Work out the finished part from the listing and answer in its coordinate system (mm). Face numbers are marked on the shaded views. A direction names the side the tool comes from. Round coordinates to 2 decimals unless told otherwise and drop trailing zeros. Order: outer loops, then holes, each group sorted by start corner. A loop starts at its lowest first (then second) coordinate and runs counter-clockwise, first axis right, second up. Notation, with made-up numbers: M 67,80 L 101,80 A26 cw 101,100 Z; hole C 68.5,-3.75 d3. An arc over 180 degrees is marked long. Answer as a JSON object with one key per item and string values. Group by question number.
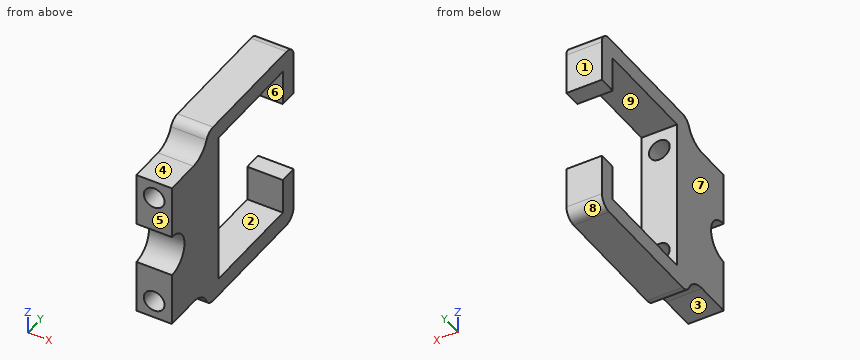
Autodesk Inventor part; units mm, degrees
ref_plane "YZ Plane" through (0, 0, 0) normal (1, 0, 0) x (0, 1, 0)
ref_plane "XZ Plane" through (0, 0, 0) normal (0, 1, 0) x (-1, 0, 0)
ref_plane "XY Plane" through (0, 0, 0) normal (0, 0, 1) x (1, 0, 0)
sketch "Esquisse1" plane through (0, 0, 0) normal (1, 0, 0) x (0, 1, 0)
  arc A0 (0, -3.5) -> (0, 3.5) centre (0, 0) ccw
  line L0 (0, 6.2947) -> (0, -6.5718) construction
  line L1 (0, 3.5) -> (0, 12.5)
  line L2 (0, 12.5) -> (10, 12.5)
  line L3 (10, -12.5) -> (0, -12.5)
  line L4 (0, -12.5) -> (0, -3.5)
  line L5 (10, 12.5) -> (10, 16)
  line L6 (10, 16) -> (34, 16)
  line L7 (34, 16) -> (34, 7)
  line L8 (34, 7) -> (31, 7)
  line L9 (31, 7) -> (31, 13)
  line L10 (31, 13) -> (13, 13)
  line L11 (13, 13) -> (13, -13)
  line L12 (13, -13) -> (31, -13)
  line L13 (31, -13) -> (31, -7)
  line L14 (31, -7) -> (34, -7)
  line L15 (34, -7) -> (34, -16)
  line L16 (34, -16) -> (10, -16)
  line L17 (10, -16) -> (10, -12.5)
  point P0 (22, 13)
  dimension "d16" = 3.5
  dimension "d17" = 25
  dimension "d18" = 26
  dimension "d19" = 6
  dimension "d20" = 3
  dimension "d21" = 3
  dimension "d22" = 3
  dimension "d23" = 18
  dimension "d24" = 3
  dimension "d25" = 10
extrude "Extrusion1" add sketch "Esquisse1" along normal blind 6
fillet "Congé1" radius 4 2 edges at (3, 10, 12.5) (3, 10, -12.5)
fillet "Congé2" radius 2 2 edges at (3, 10, -16) (3, 10, 16)
fillet "Congé3" radius 2 2 edges at (3, 34, 16) (3, 34, -16)
sketch "Esquisse2" plane through (0, 0, -12.5) normal (0, -1, 0) x (1, 0, 0)
  circle A0 centre (3, 3) radius 1.75
  line L0 (0, -1.5) -> (0, 5.5)
  line L1 (6, -0.5) -> (6, 25.5)
  line L2 (0, -0.5) -> (0, 25.5)
  line L3 (0, 0) -> (6, 0)
  point P0 (0, 12.5)
  point P1 (3, 3)
  dimension "d28" = 3.5
  dimension "d31" = 3
  dimension "d32" = 3
extrude "Extrusion2" cut sketch "Esquisse2" against normal blind 15
mirror "Mise en miroir1" about plane through (0, 0, 0) normal (0, 0, 1) of "Extrusion2"
properties part number "Bras_1_Impression 3D"
Item 1: Each of these flat-tipped pins is pushed along its axis until it touches: pin 1 (1.8 mm diameter, centred on x = 3.5, y = 4, fed in from +Z); pin 2 (1.5 mm diameter, centred on x = 2, y = 33, fed in from +Z); pin 3 (1.8 mm diameter, centred on x = 3, y = 1.5, fed in from -Z). Where does it stop, or does it pass through?
Item 2: Consider L1, parallel to Z at x = 3, y = 6; L2, parallel to Z at x = 3.45, y = 14.5; L3, parallel to X at y = 5.25, z = 9.5. Determine where each line is inside the solid, lowest interval first.
Item 3: Find section A-A (z = -9.5). Give the vertices of the cut face in (x, y), and give its area (3 significant figures).
Item 4: A tool of negligible diameter and unlimited length cuts with its end or side. For the marked faces 1, 2, 3, 4 and 5, from which of +Z, -Z, +X, -X, +Y, -Y can it reach the whole face along a straight path? Write none if from no direction.
Item 5: Find section C-C (y = 27). Give the vertices of the cut face in (x, z).
Item 6: The mould has two halves that part along Z. Classify the marked faces 6, 7, 8 and 9: +Z half, -Z half, draft (parallel to the pull), parting line (faces both ways), or undercut.
Item 7: Find section B-B (x = 3). Give the number of separate pieces and of enclosed holes in the cut face, and give its area (3 significant figures).
Item 8: Find section D-D (x = 0.45). Give the vertices of the cut face in (y, z).
Responses:
{
 "1": {"pin 1": "stops at z = 12.5", "pin 2": "stops at z = 15.98", "pin 3": "stops at z = -12.5"},
 "2": {"L1": "z = -12.5 to -11.25, -7.75 to 7.75, 11.25 to 12.5", "L2": "z = -16 to -13, 13 to 16", "L3": "x = 0 to 1.25, 4.75 to 6"},
 "3": {"outline": "M 0,0 L 1.25,0 L 1.25,13 L 0,13 Z; M 0,31 L 6,31 L 6,34 L 0,34 Z; M 4.75,0 L 6,0 L 6,13 L 4.75,13 Z", "area": "50.5 mm^2"},
 "4": {"face 1": "+Z, -Z, +X, -X, +Y", "face 2": "+X, -X", "face 3": "-Z, +X, -X, -Y", "face 4": "+Z, +X, -X, -Y", "face 5": "+Z, -Z, +X, -X, -Y"},
 "5": {"outline": "M 0,-16 L 6,-16 L 6,-13 L 0,-13 Z; M 0,13 L 6,13 L 6,16 L 0,16 Z"},
 "6": {"face 6": "undercut", "face 7": "draft", "face 8": "-Z half", "face 9": "undercut"},
 "7": {"separate pieces": "3", "enclosed holes": "0", "area": "402 mm^2"},
 "8": {"outline": "M 0,-12.5 L 6.03,-12.5 A4 cw 9.67,-14.83 A2 ccw 11.49,-16 L 32,-16 A2 ccw 34,-14 L 34,-7 L 31,-7 L 31,-13 L 13,-13 L 13,13 L 31,13 L 31,7 L 34,7 L 34,14 A2 ccw 32,16 L 11.49,16 A2 ccw 9.67,14.83 A4 cw 6.03,12.5 L 0,12.5 L 0,3.5 A3.5 cw 0,-3.5 Z"}
}
